Design review of the part built by this model. Coordinates are the model's own, in mm. A direction names the side the tool comes from. Coordinates: 2 decimals unless noted, no trailing zeros. Write each loop counter-clockwise with the first axis right and the second up, starting at its lowest first coordinate (ties: lowest second). Pieces come first, ordered by that corner, then holes. Notation, with made-up numbers: (46.25, 85.25) -> (50.25, 85.25) arc R16 cw to (50.25, 98.25) -> close; hole circle Ø1 at (-25, 15.25). An arc over 180 degrees is marked (long way). Answer in a Markdown table with one row per item. Add a question column.
Item 1: Take a section at C-C, the plane z = 115.5. Write out the cut boundary in (x, y), and give its area (3 significant figures).
Item 2: Take a section at B-B, the plane y = 8.5. Write out the cut boundary in (x, z), and give its area (3 significant figures).
Item 3: For faces 4 (the face through (47, 8, 4)), 5 (the face through (0, 7, 272)), list the 3-axis set-ups (+Z, -Z, +X, -X, +Y, -Y) from which the entire face can be reached by the end or side of a thin tool; tool diameter is ignored.
Item 4: Clearance check with flat-ended pins moving along their axes: P1, Ø5.5, axis at x = 64, z = 269.5, coming from the -Y side; P2, Ø3, axis at y = 4.5, z = 154, coming from the -X side. State where each tip first meets the part, or that it passes through.
Item 5: To check wall thickness, follow line 1 (Z direction, x = 32.5, y = 8); line 2 (Z direction, x = 34, y = 13.5); line 3 (X direction, y = 2.75, z = 151). State the ranges of each line that lie inside material, in increasing order.
Item 6: Draft analysis for pull direction Y (two halves, no side actions). For faces 1 (the face through (98, 15, 138)), 2 (the face through (49, 8, 0)), 3 (the face through (47, 2.5, 6)), state which applies: released by +Y, released by -Y, zero draft, split by the parting line, or undercut.
Item 7: Take a section at A-A, the plane x = 74. Write out the cut boundary in (y, z).
from build123d import *

# Parameters (mm, degrees)
ESQUISSE1_W        = 100
ESQUISSE1_H        = 15
BOSS_EXTRU_1_DEPTH = 4
ESQUISSE2_W        = 100
ESQUISSE2_H        = 2.5
BOSS_EXTRU_2_DEPTH = 5
ESQUISSE3_W        = 5
ESQUISSE3_H        = 15
BOSS_EXTRU_3_DEPTH = 267.12


with BuildPart() as part:
    # Esquisse1 → Boss.-Extru.1 (new body)
    with BuildSketch(Plane.XY):
        with Locations((50, 7.5)):
            Rectangle(ESQUISSE1_W, ESQUISSE1_H)
    boss_extru_1 = extrude(amount=BOSS_EXTRU_1_DEPTH)

    # Esquisse2 → Boss.-Extru.2 (add)
    with BuildSketch(Plane.XY.offset(4)):
        with Locations((50, 13.75)):
            Rectangle(ESQUISSE2_W, ESQUISSE2_H)
        with Locations((50, 1.25)):
            Rectangle(ESQUISSE2_W, ESQUISSE2_H)
    boss_extru_2 = extrude(amount=BOSS_EXTRU_2_DEPTH)

    # Esquisse3 → Boss.-Extru.3 (add)
    with BuildSketch(Plane.XY.offset(4)):
        with Locations((97.5, 7.5)):
            Rectangle(ESQUISSE3_W, ESQUISSE3_H)
    extrude(amount=BOSS_EXTRU_3_DEPTH)

    # Symétrie2: Boss.-Extru.1, Boss.-Extru.2 across plane
    add(boss_extru_1.mirror(Plane.XY.offset(137.56)))
    add(boss_extru_2.mirror(Plane.XY.offset(137.56)))


solid = part.part
Answers:
| question | item | result |
|---|---|---|
| 1 | outline | (95, 0) -> (100, 0) -> (100, 15) -> (95, 15) -> close |
| 1 | area | 75.0 mm^2 |
| 2 | outline | (0, 0) -> (100, 0) -> (100, 275.12) -> (0, 275.12) -> (0, 271.12) -> (95, 271.12) -> (95, 4) -> (0, 4) -> close |
| 2 | area | 2,140 mm^2 |
| 3 | face 4 | -X |
| 3 | face 5 | +Z, -Z, -X, +Y, -Y |
| 4 | P1 | stops at y = 0 |
| 4 | P2 | stops at x = 95 |
| 5 | line 1 | z = 0 to 4, 271.12 to 275.12 |
| 5 | line 2 | z = 0 to 9, 266.12 to 275.12 |
| 5 | line 3 | x = 95 to 100 |
| 6 | face 1 | released by +Y |
| 6 | face 2 | zero draft |
| 6 | face 3 | undercut |
| 7 | outline | (0, 0) -> (15, 0) -> (15, 9) -> (12.5, 9) -> (12.5, 4) -> (2.5, 4) -> (2.5, 9) -> (0, 9) -> close; (0, 266.12) -> (2.5, 266.12) -> (2.5, 271.12) -> (12.5, 271.12) -> (12.5, 266.12) -> (15, 266.12) -> (15, 275.12) -> (0, 275.12) -> close |
